For this review, use the dimensioned drawing (mm, ordinates from the lowest corner) and the shaded views. Give positions to 0.01 mm unless a question says otherwise; leave off trailing zeros. Loops run counter-clockwise (first coordinate to the right, second up) from the corner with the lowest first, then second, coordinate; pieces in that order, holes last. Notation, with made-up numbers: (51.25, 8.5) -> (79.25, 8.5) arc R37 cw to (79.25, 47.5) -> close; hole circle Ø3 at (43, 5.5). An arc over 180 degrees is marked (long way). Write each question's results on one line, items separated by ' | '. Start each with the question number.
Q1. We need section D-D (z = 6.5). Write out the cut boundary in (x, y).
Q2. Wall thickness on L1, parallel to X at y = 1.1, z = 13; L2, parallel to Z at x = 6, y = 1.25 (1 decimal); L3, parallel to X at y = 1.25, z = 18.5 (1 decimal): over which ranges is each line inside the solid? List them lowest first. Write a range as [from, to].
Q3. We need section A-A (z = 13). Write out the cut boundary in (x, y), plus the area to 3 significant figures.
Q4. We need section C-C (y = 0.65). Write out the cut boundary in (x, z).
Q5. We need section B-B (x = 6.5). Write out the cut boundary in (y, z).
Q6. Insertion check: pin 1 Ø1.8 at (x, z) = (6.5, 19) entering from -Y. The pin has a flat end and moves straight along its axis. Give the tip position at first contact, or say it passes through.
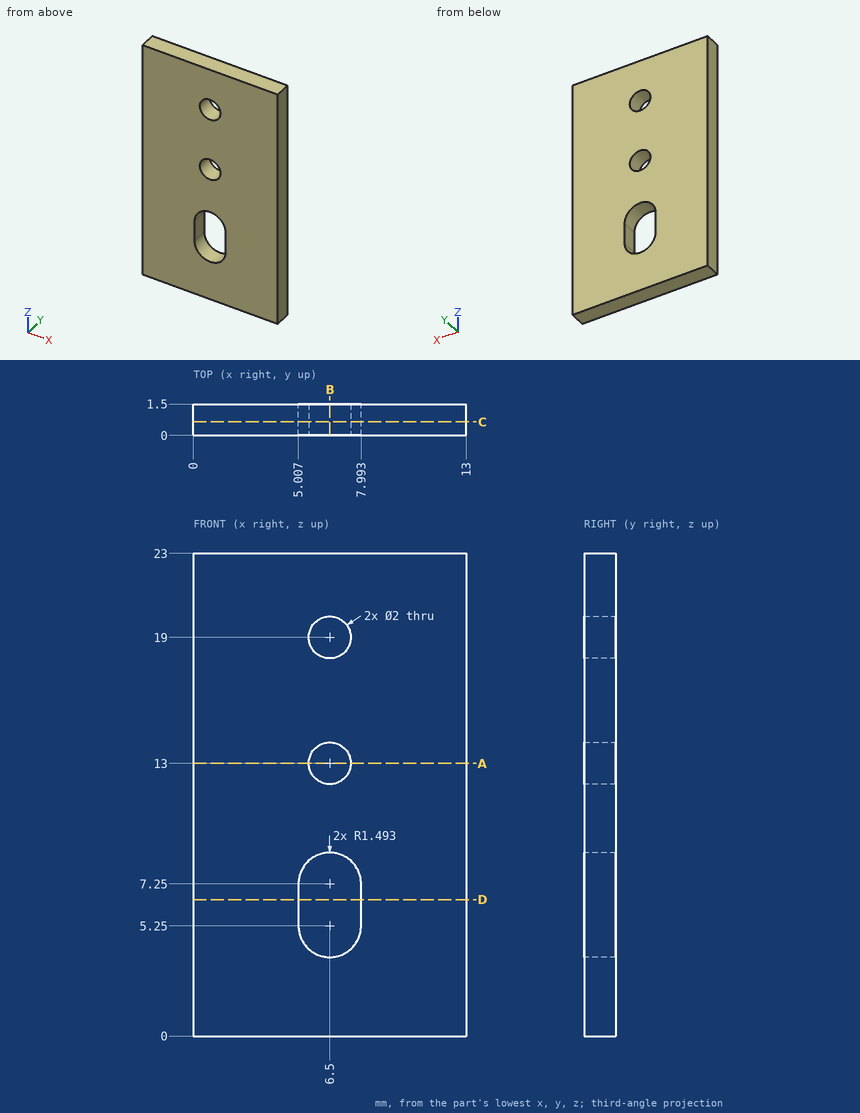
Output:
1) outline: (0, 0) -> (5.01, 0) -> (5.01, 1.5) -> (0, 1.5) -> close; (7.99, 0) -> (13, 0) -> (13, 1.5) -> (7.99, 1.5) -> close
2) L1: [0, 5.5], [7.5, 13] | L2: [0, 3.8], [8.7, 12.1], [13.9, 18.1], [19.9, 23] | L3: [0, 5.6], [7.4, 13]
3) outline: (0, 0) -> (5.5, 0) -> (5.5, 1.5) -> (0, 1.5) -> close; (7.5, 0) -> (13, 0) -> (13, 1.5) -> (7.5, 1.5) -> close | area: 16.5 mm2
4) outline: (0, 0) -> (13, 0) -> (13, 23) -> (0, 23) -> close; hole (5.01, 5.25) arc R1.49 ccw to (7.99, 5.25) -> (7.99, 7.25) arc R1.49 ccw to (5.01, 7.25) -> close; hole circle Ø2 at (6.5, 13); hole circle Ø2 at (6.5, 19)
5) outline: (0, 0) -> (1.5, 0) -> (1.5, 3.76) -> (0, 3.76) -> close; (0, 8.74) -> (1.5, 8.74) -> (1.5, 12) -> (0, 12) -> close; (0, 14) -> (1.5, 14) -> (1.5, 18) -> (0, 18) -> close; (0, 20) -> (1.5, 20) -> (1.5, 23) -> (0, 23) -> close
6) pin 1: through
